Design review of the part shown in the three views and the two pictorial views. Dimensions are in mm from the part's minimum x, y and z. Coordinates: 2 decimals unless noted, no trailing zeros. Write each loop counter-clockwise with the first axis right and the second up, starting at its lowest first coordinate (ties: lowest second). Pieces come first, ordered by that corner, then holes. Notation, with made-up numbers: (70.5, 88) -> (118.5, 88) arc R17 cw to (118.5, 113) -> close; hole circle Ø1 at (41.5, 48.25). An arc over 180 degrees is marked (long way). Answer in a Markdown table with one row per item. Add a question column.
Item 1: Take a section at D-D, the plane x = 50.5. Write out the cut boundary in (y, z).
Item 2: To check wall thickness, follow line 1 (Y direction, x = 38.5, z = 1.05); line 2 (X direction, y = 33, z = 1.7); line 3 (X direction, y = 4, z = 0.7). State the ranges of each line that lie inside material, in increasing order.
Item 3: Take a section at C-C, the plane y = 18. Write out the cut boundary in (x, z).
Item 4: Clearance check with flat-ended pins moving along their axes: P1, Ø1.5, axis at x = 18, z = 2, coming from the +Y side; P2, Ø0.9, axis at y = 28, z = 1, coming from the +X side; P3, Ø1.5, axis at x = 30, z = 1.5, coming from the -Y side. State where each tip first meets the part, or that it passes through.
Item 5: Take a section at B-B, the plane z = 2.1. Give the number of separate pieces and of enclosed holes in the cut face.
Item 6: Take a section at A-A, the plane y = 22. Write out the cut boundary in (x, z).
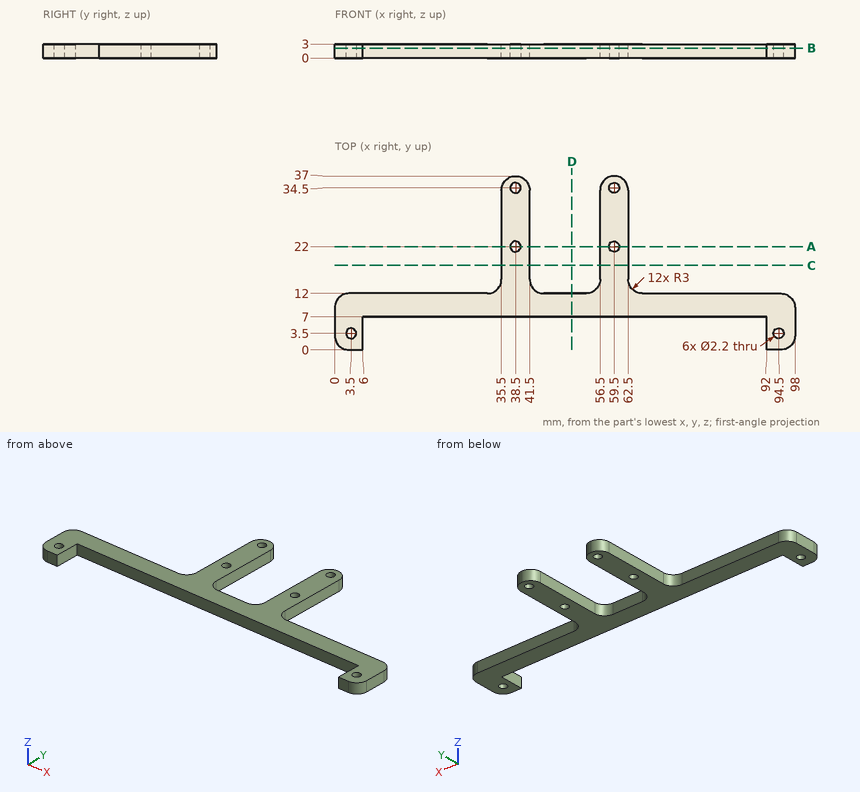
Answers:
| question | item | result |
|---|---|---|
| 1 | outline | (7, 0) -> (12, 0) -> (12, 3) -> (7, 3) -> close |
| 2 | line 1 | y = 7 to 20.9, 23.1 to 33.4, 35.6 to 37 |
| 2 | line 2 | x = 35.5 to 41.5, 56.5 to 62.5 |
| 2 | line 3 | x = 0 to 2.52, 4.48 to 6, 92 to 93.52, 95.48 to 98 |
| 3 | outline | (35.5, 0) -> (41.5, 0) -> (41.5, 3) -> (35.5, 3) -> close; (56.5, 0) -> (62.5, 0) -> (62.5, 3) -> (56.5, 3) -> close |
| 4 | P1 | stops at y = 12 |
| 4 | P2 | stops at x = 62.5 |
| 4 | P3 | stops at y = 7 |
| 5 | separate pieces | 1 |
| 5 | enclosed holes | 6 |
| 6 | outline | (35.5, 0) -> (37.4, 0) -> (37.4, 3) -> (35.5, 3) -> close; (39.6, 0) -> (41.5, 0) -> (41.5, 3) -> (39.6, 3) -> close; (56.5, 0) -> (58.4, 0) -> (58.4, 3) -> (56.5, 3) -> close; (60.6, 0) -> (62.5, 0) -> (62.5, 3) -> (60.6, 3) -> close |
